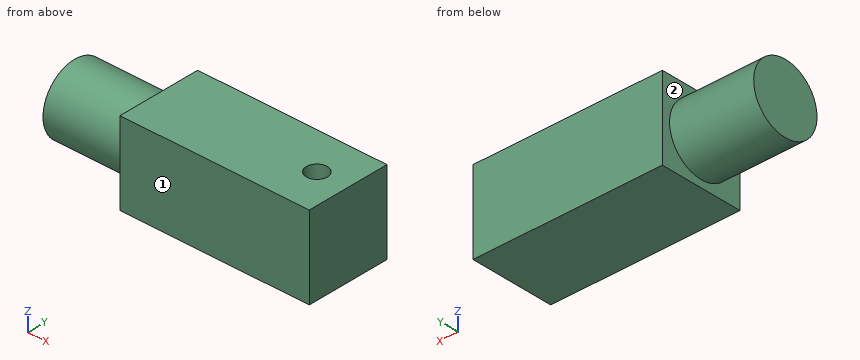
from build123d import *

# Parameters (mm, degrees)
SKETCH1_W           = 45.72
SKETCH1_H           = 20
BOSS_EXTRUDE1_DEPTH = 20.32
SKETCH2_R           = 8.276149927
BOSS_EXTRUDE2_DEPTH = 20.32
SKETCH4_R           = 2.54
CUT_EXTRUDE1_DEPTH  = 19.05


with BuildPart() as part:
    # Sketch1 → Boss-Extrude1 (new body)
    with BuildSketch(Plane(origin=(0, 0, 1.285201824), x_dir=(1, 0, 0), z_dir=(0, 1, 0))):
        with Locations((-5.388735632, 10)):
            Rectangle(SKETCH1_W, SKETCH1_H)
    extrude(amount=BOSS_EXTRUDE1_DEPTH)

    # Sketch2 → Boss-Extrude2 (add)
    with BuildSketch(Plane(origin=(-28.248735632, 0, 1.285201824), x_dir=(0, 0, 1), z_dir=(-1, 0, 0))):
        with Locations((-10, 10.16)):
            Circle(SKETCH2_R)
    extrude(amount=BOSS_EXTRUDE2_DEPTH)

    # Sketch4 → Cut-Extrude1 (cut)
    with BuildSketch(Plane.XY.offset(1.285201824)):
        with Locations((9.928717344, 10.16)):
            Circle(SKETCH4_R)
    extrude(amount=-CUT_EXTRUDE1_DEPTH, mode=Mode.SUBTRACT)


solid = part.part
Geometry: final body of the model. Coordinates: model frame, mm. Face numbers are marked on the shaded views. A direction names the side the tool comes from. Round coordinates to 2 decimals unless told otherwise and drop trailing zeros. Order: outer loops, then holes, each group sorted by start corner. A loop starts at its lowest first (then second) coordinate and runs counter-clockwise, first axis right, second up.
Q1. Access query for the marked faces 1 and 2. Directions: +Z, -Z, +X, -X, +Y, -Y. A direction counts if a zero-diameter tool reaches every point of the face in a straight line with its end or side. Return the directions, or none.
Result sheet:
face 1: +Z, -Z, +X, -X, -Y
face 2: -X
Q2. Section D-D, the plane y = 15.25. Output: boundary loops of the cut face in (x, z), and give its area (3 significant figures).
Result sheet:
outline: (-48.57, -15.24) - (-28.25, -15.24) - (-28.25, -18.71) - (17.47, -18.71) - (17.47, 1.29) - (-28.25, 1.29) - (-28.25, -2.19) - (-48.57, -2.19) - close
area: 1,180 mm2
Q3. Section B-B, the plane x = 8. Output: boundary loops of the cut face in (y, z), and give its area (3 significant figures).
Result sheet:
outline: (0, -18.71) - (20.32, -18.71) - (20.32, 1.29) - (11.81, 1.29) - (11.81, -17.76) - (8.51, -17.76) - (8.51, 1.29) - (0, 1.29) - close
area: 343 mm2
Q4. Section C-C, the plane x = -31.5. Output: boundary loops of the cut face in (y, z), and give its area (3 significant figures).
Result sheet:
outline: circle Ø16.55 at (10.16, -8.71)
area: 215 mm2
Q5. Material intervals for probe 1 along Z at (x, y) = (9, 8.25); probe 2 along X at (y, z) = (10.5, -8.75); probe 3 along X at (y, z) = (18, -15.75), sorted ascending.
Result sheet:
probe 1: z = -18.71 to -17.76
probe 2: x = -48.57 to 7.41, 12.45 to 17.47
probe 3: x = -28.25 to 17.47
Q6. Section A-A, the plane y = 10.16. Output: boundary loops of the cut face in (x, z), and give its area (3 significant figures).
Result sheet:
outline: (-48.57, -16.99) - (-28.25, -16.99) - (-28.25, -18.71) - (17.47, -18.71) - (17.47, 1.29) - (12.47, 1.29) - (12.47, -17.76) - (7.39, -17.76) - (7.39, 1.29) - (-28.25, 1.29) - (-28.25, -0.44) - (-48.57, -0.44) - close
area: 1,150 mm2
Q7. Pin query (flat end, axial travel): pin 1 (4 mm diameter, centred on x = -21.5, z = -5, fed in from -Y); pin 2 (1.5 mm diameter, centred on x = 9.5, y = 11.5, fed in from +Z). Return the tip coordinate at first contact, or that it passes through.
Result sheet:
pin 1: stops at y = 0
pin 2: stops at z = -17.76
